The listing builds one solid part. Answer for the finished solid, in the listing's coordinates (mm). A direction names the side the tool comes from. Coordinates: 2 decimals unless noted, no trailing zeros. Loops run counter-clockwise (first coordinate to the right, second up) from the corner with the lowest first, then second, coordinate; pieces in that order, holes last. Notation, with made-up numbers: M 51.25,80.5 L 78.25,80.5 A33 cw 78.25,111.5 Z; hole C 82.25,71 d6. An arc over 180 degrees is marked long. Answer as a JSON object with one key per item and string values. Group by question number.
1. Straight lines are drawn through the part: L1, parallel to X at y = 6.25, z = -50.5 (3 decimals); L2, parallel to X at y = 9.5, z = -50.5 (3 decimals); L3, parallel to X at y = 6.35, z = -5. For each, find the intervals that lie inside material, in ascending order.
2. A cutting plane is placed at B-B on z = -50.5. Give the vertices of the cut face in (x, y) (3 decimals), and give its area (3 significant figures).
3. A cutting plane is placed at A-A on y = 4. Give the vertices of the cut face in (x, z) (3 decimals).
4. A cutting plane is placed at D-D on y = 10.75. Give the vertices of the cut face in (x, z) (3 decimals), and give its area (3 significant figures).
5. A cutting plane is placed at C-C on x = 15. Give the vertices of the cut face in (y, z), and give its area (3 significant figures).
6. Given pin 1 (8.5 mm diameter, centred on x = 22.5, y = 14.5, fed in from +Z); pin 2 (5 mm diameter, centred on y = 14, z = -16.5, fed in from -X); pin 3 (3 mm diameter, centred on x = 36, z = -51.5, fed in from +Y), each flat-ended and moving along its own axis, determine where each tip first touches the part or whether it passes through.
7. For faces 5 (the face through (35, 14.9, -48.5)), 6 (the face through (34, 7, -15)), 7 (the face through (30.9, 1.479, -18.787)), determine the directions among +Z, -Z, +X, -X, +Y, -Y from which every point of the face is accessible in a straight line to the end or side of a thin tool.
8. Determine the mould class of faces 1 (the face through (23, 3, 0)), 2 (the face through (0, 5, -37)), 3 (the face through (13.2, 16.5, -52.9)), 4 (the face through (34.33, 7.554, -48.883)) for opening direction X: released by +X, released by -X, zero draft, split by the parting line, or undercut.
from build123d import *

# Parameters (mm, degrees)
OUTLINESKETCH2_W                               = 50
OUTLINESKETCH2_H                               = 61
OUTLINESKETCH2_R                               = 2
OUTLINEBOSS_EXTRUDE1_DEPTH                     = 18
BUILDPLATECUTOUTSKETCH1_W                      = 49
BUILDPLATECUTOUTSKETCH1_H                      = 46
BUILDPLATECUTOUTCUT_EXTRUDE7_DEPTH             = 10.5
HEATMATCUTSKETCH3_W                            = 34
HEATMATCUTSKETCH3_H                            = 31
HEATMATCUT_EXTRUDE8_DEPTH                      = 2
BALLJOINTCUT_EXTRUDE9_DEPTH                    = 3
SKETCH1_R                                      = 1.75
SKETCH1_R_2                                    = 2.675
ZENDSTOPSWITCHMOUNTHOLESCUT_EXTRUDE1_DEPTH     = 81.901174281
SKETCH3_R                                      = 3
ZENDSTOPSWITCHMOUNTBOREHOLESCUT_EXTRUDE2_DEPTH = 3.1
SKETCH4_R                                      = 4.125
ZENDSTOPSWITCHCONNINGTOWERTBORECUT_EXTRU_DEPTH = 7.5


with BuildPart() as part:
    # OutlineSketch2 → OutlineBoss-Extrude1 (new body)
    with BuildSketch(Plane(origin=(0, 0, 0), x_dir=(1, 0, 0), z_dir=(0, 1, 0))):
        with Locations((25, 30.5)):
            Rectangle(OUTLINESKETCH2_W, OUTLINESKETCH2_H)
        with Locations(Location((42, 5, 0), (0, 0, 270))):
            Circle(OUTLINESKETCH2_R, mode=Mode.SUBTRACT)
    extrude(amount=OUTLINEBOSS_EXTRUDE1_DEPTH)

    # BuildPlateCutoutSketch1 → BuildPlateCutoutCut-Extrude7 (cut)
    with BuildSketch(Plane(origin=(0, 18, 0), x_dir=(1, 0, 0), z_dir=(0, 1, 0))):
        with Locations((24.5, 23)):
            Rectangle(BUILDPLATECUTOUTSKETCH1_W, BUILDPLATECUTOUTSKETCH1_H)
    extrude(amount=-BUILDPLATECUTOUTCUT_EXTRUDE7_DEPTH, mode=Mode.SUBTRACT)

    # HeatMatCutSketch3 → HeatMatCut-Extrude8 (cut)
    with BuildSketch(Plane(origin=(0, 7.5, 0), x_dir=(1, 0, 0), z_dir=(0, 1, 0))):
        with Locations((17, 15.5)):
            Rectangle(HEATMATCUTSKETCH3_W, HEATMATCUTSKETCH3_H)
    extrude(amount=-HEATMATCUT_EXTRUDE8_DEPTH, mode=Mode.SUBTRACT)

    # BallJointCutoutSketch4 → BallJointCut-Extrude9 (cut)
    with BuildSketch(Plane.XZ):
        with BuildLine():
            Line((25.020895194, 0), (50, 0))
            Line((50, 0), (50, -20.788920166))
            ThreePointArc((50, -20.788920166), (30.677417203, -18.604746187), (25.020895194, 0))
        make_face()
    extrude(amount=-BALLJOINTCUT_EXTRUDE9_DEPTH, mode=Mode.SUBTRACT)

    # Sketch1 → ZEndStopSwitchMountHolesCut-Extrude1 (cut, through all)
    with BuildSketch(Plane(origin=(0, 18, 0), x_dir=(1, 0, 0), z_dir=(0, 1, 0))):
        with Locations(Location((35, 50.5, 0), (0, 0, 270))):
            Circle(SKETCH1_R)
        with Locations(Location((25, 50.5, 0), (0, 0, 270))):
            Circle(SKETCH1_R_2)
        with Locations(Location((15, 50.5, 0), (0, 0, 270))):
            Circle(SKETCH1_R)
    extrude(amount=-ZENDSTOPSWITCHMOUNTHOLESCUT_EXTRUDE1_DEPTH, mode=Mode.SUBTRACT)

    # Sketch3 → ZEndStopSwitchMountBoreHolesCut-Extrude2 (cut)
    with BuildSketch(Plane(origin=(0, 18, 0), x_dir=(1, 0, 0), z_dir=(0, 1, 0))):
        with Locations(Location((35, 50.5, 0), (0, 0, 270))):
            Circle(SKETCH3_R)
        with Locations(Location((15, 50.5, 0), (0, 0, 270))):
            Circle(SKETCH3_R)
    extrude(amount=-ZENDSTOPSWITCHMOUNTBOREHOLESCUT_EXTRUDE2_DEPTH, mode=Mode.SUBTRACT)

    # Sketch4 → ZEndStopSwitchConningTowertBoreCut-Extrude1 (cut)
    with BuildSketch(Plane.XZ):
        with Locations(Location((25, -50.5, 0), (0, 0, 270))):
            Circle(SKETCH4_R)
    extrude(amount=-ZENDSTOPSWITCHCONNINGTOWERTBORECUT_EXTRU_DEPTH, mode=Mode.SUBTRACT)


solid = part.part
From the geometry:
{
 "1": {"L1": "x = 0 to 13.25, 16.75 to 20.875, 29.125 to 33.25, 36.75 to 50", "L2": "x = 0 to 13.25, 16.75 to 22.325, 27.675 to 33.25, 36.75 to 50", "L3": "x = 34 to 40, 44 to 50"},
 "2": {"outline": "M 0,0 L 13.25,0 L 13.25,14.9 L 12,14.9 L 12,18 L 0,18 Z; M 16.75,0 L 20.875,0 L 20.875,7.5 L 22.325,7.5 L 22.325,18 L 18,18 L 18,14.9 L 16.75,14.9 Z; M 27.675,7.5 L 29.125,7.5 L 29.125,0 L 33.25,0 L 33.25,14.9 L 32,14.9 L 32,18 L 27.675,18 Z; M 36.75,0 L 50,0 L 50,18 L 38,18 L 38,14.9 L 36.75,14.9 Z", "area": "640 mm²"},
 "3": {"outline": "M 0,-61 L 50,-61 L 50,0 L 0,0 Z; hole C 15,-50.5 d3.5; hole C 25,-50.5 d8.25; hole C 35,-50.5 d3.5; hole C 42,-5 d4"},
 "4": {"outline": "M 0,-61 L 50,-61 L 50,0 L 49,0 L 49,-46 L 0,-46 Z; hole C 15,-50.5 d3.5; hole C 25,-50.5 d5.35; hole C 35,-50.5 d3.5", "area": "754 mm²"},
 "5": {"outline": "M 0,-61 L 18,-61 L 18,-53.5 L 14.9,-53.5 L 14.9,-52.25 L 0,-52.25 Z; M 0,-48.75 L 14.9,-48.75 L 14.9,-47.5 L 18,-47.5 L 18,-46 L 7.5,-46 L 7.5,-31 L 5.5,-31 L 5.5,0 L 0,0 Z", "area": "482 mm²"},
 "6": {"pin 1": "stops at z = -46", "pin 2": "stops at x = 49", "pin 3": "stops at y = 14.9"},
 "7": {"face 5": "+Y", "face 6": "+Z, -X, +Y", "face 7": "-Y"},
 "8": {"face 1": "zero draft", "face 2": "released by -X", "face 3": "undercut", "face 4": "undercut"}
}
